```python
from build123d import *

# Parameters (mm, degrees)
SKETCH1_W           = 129.9464
SKETCH1_H           = 120.8024
BOSS_EXTRUDE1_DEPTH = 5.7912
SKETCH3_W           = 43.315466666
SKETCH3_H           = 5.7912
CUT_EXTRUDE2_DEPTH  = 89.900841825
SKETCH6_W           = 5.7912
SKETCH6_H           = 40.267466666
CUT_EXTRUDE5_DEPTH  = 89.900841825
SKETCH7_W           = 13.7668
SKETCH7_H           = 2.6035
CUT_EXTRUDE6_DEPTH  = 89.900841825
SKETCH8_W           = 2.0828
SKETCH8_H           = 6.1722
CUT_EXTRUDE7_DEPTH  = 89.900841825
CAVITY1_START       = -64.9732
CAVITY1_OUTLINE_W   = 40.267466667
CAVITY1_OUTLINE_H   = 5.7912
CAVITY1_DEPTH       = 5.7912
CAVITY1_START_2     = 21.657733333
CAVITY1_2_OUTLINE_W = 5.7912
CAVITY1_2_OUTLINE_H = 5.7912
CAVITY1_2_DEPTH     = 43.315466667
CAVITY1_START_3     = -59.182
CAVITY1_3_OUTLINE_W = 5.7912
CAVITY1_3_OUTLINE_H = 5.7912
CAVITY1_3_DEPTH     = 37.524266667


# Read off the part's stored shape, not the designer's step: Cavity1
with BuildPart() as part:
    # Sketch1 → Boss-Extrude1 (new body)
    with BuildSketch(Plane.XY):
        Rectangle(SKETCH1_W, SKETCH1_H)
    extrude(amount=BOSS_EXTRUDE1_DEPTH)

    # Sketch3 → Cut-Extrude2 (cut, through all)
    with BuildSketch(Plane(origin=(0, 0, 0), x_dir=(-1, 0, 0), z_dir=(0, 0, -1))):
        with Locations((0, -57.5056)):
            Rectangle(SKETCH3_W, SKETCH3_H)
    extrude(amount=-CUT_EXTRUDE2_DEPTH, mode=Mode.SUBTRACT)

    # Sketch6 → Cut-Extrude5 (cut, through all)
    with BuildSketch(Plane(origin=(0, 0, 0), x_dir=(-1, 0, 0), z_dir=(0, 0, -1))):
        with Locations((-62.0776, 0)):
            Rectangle(SKETCH6_W, SKETCH6_H)
    extrude(amount=-CUT_EXTRUDE5_DEPTH, mode=Mode.SUBTRACT)

    # Sketch7 → Cut-Extrude6 (cut, through all)
    with BuildSketch(Plane(origin=(0, 0, 0), x_dir=(-1, 0, 0), z_dir=(0, 0, -1))):
        with Locations((-52.2986, 0)):
            Rectangle(SKETCH7_W, SKETCH7_H)
    extrude(amount=-CUT_EXTRUDE6_DEPTH, mode=Mode.SUBTRACT)

    # Sketch8 → Cut-Extrude7 (cut, through all)
    with BuildSketch(Plane(origin=(0, 0, 0), x_dir=(-1, 0, 0), z_dir=(0, 0, -1))):
        with Locations((-52.2986, 0)):
            Rectangle(SKETCH8_W, SKETCH8_H)
    extrude(amount=-CUT_EXTRUDE7_DEPTH, mode=Mode.SUBTRACT)

    # Cavity1 outline → Cavity1 (cut)
    with BuildSketch(Plane.YZ.offset(CAVITY1_START)):
        with Locations((40.267466666, 2.8956)):
            Rectangle(CAVITY1_OUTLINE_W, CAVITY1_OUTLINE_H)
        with Locations((-40.267466666, 2.8956)):
            Rectangle(CAVITY1_OUTLINE_W, CAVITY1_OUTLINE_H)
    extrude(amount=CAVITY1_DEPTH, mode=Mode.SUBTRACT)

    # Cavity1 2 outline → Cavity1 2 (cut)
    with BuildSketch(Plane.YZ.offset(CAVITY1_START_2)):
        with Locations((57.5056, 2.8956)):
            Rectangle(CAVITY1_2_OUTLINE_W, CAVITY1_2_OUTLINE_H)
    extrude(amount=CAVITY1_2_DEPTH, mode=Mode.SUBTRACT)

    # Cavity1 3 outline → Cavity1 3 (cut)
    with BuildSketch(Plane.YZ.offset(CAVITY1_START_3)):
        with Locations((57.5056, 2.8956)):
            Rectangle(CAVITY1_3_OUTLINE_W, CAVITY1_3_OUTLINE_H)
    extrude(amount=CAVITY1_3_DEPTH, mode=Mode.SUBTRACT)


solid = part.part
```
Could you check a few things on this model? Use its own coordinates, in mm. A direction names the side the tool comes from. Round coordinates to 2 decimals unless told otherwise and drop trailing zeros. Loops run counter-clockwise (first coordinate to the right, second up) from the corner with the lowest first, then second, coordinate; pieces in that order, holes last. Notation, with made-up numbers: (24, 78) -> (36, 78) arc R20 cw to (36, 111) -> close; hole circle Ø4 at (-12.5, 38). An arc over 180 degrees is marked (long way). One line per question, with ' | ' between items.
(1) If I drill on probe 1 along X at (y, z) = (49, 4.4); probe 2 along Y at (x, z) = (-51.5, 4.8); probe 3 along Y at (x, z) = (-18, 1.6), over which ranges is the centre line in solid material (lowest first)?
Model answer:
probe 1: x = -59.18 to 64.97 | probe 2: y = -60.4 to 54.61 | probe 3: y = -54.61 to 60.4
(2) For pin 1 Ø1.7 at (x, z) = (-46.5, 2) entering from +Y; pin 2 Ø1.7 at (x, z) = (-62.5, 1.5) entering from -Y; pin 3 Ø8 at (x, y) = (-47.5, 21) entering from -Z; pin 4 Ø3 at (y, z) = (37.5, 3.5) entering from -X, each with a flat end and sliding along its axis, tell me the tip position at first contact or that it passes through.
Model answer:
pin 1: stops at y = 54.61 | pin 2: stops at y = -20.13 | pin 3: stops at z = 0 | pin 4: stops at x = -59.18
(3) Thinking about a two-plate mould opening in X: for faces 4 (the face through (-64.973, 0, 3)), 5 (the face through (-1, 1, 5.791)), 6 (the face through (64.973, 37, 3)), 7 (the face through (21.658, -58, 3)), which applies, released by +X, released by -X, zero draft, split by the parting line, or undercut?
Model answer:
face 4: released by -X | face 5: zero draft | face 6: released by +X | face 7: undercut
(4) If we section it at B-B on x = 36: List the corners of the cut face in (y, z) for me.
Model answer:
outline: (-60.4, 0) -> (54.61, 0) -> (54.61, 5.79) -> (-60.4, 5.79) -> close
(5) For faces 1 (the face through (-41, 54.61, 3)), 2 (the face through (0, -54.61, 3)), 3 (the face through (62, 20.134, 3)), which set-ups out of +Z, -Z, +X, -X, +Y, -Y let a thin tool reach every point of the face, with its end or its side?
Model answer:
face 1: +Z, -Z, -X, +Y | face 2: +Z, -Z, -Y | face 3: +Z, -Z, +X
(6) If we section it at C-C on y = 48: List the corners of the cut face in (x, z) for me, and give its area (3 significant figures).
Model answer:
outline: (-59.18, 0) -> (64.97, 0) -> (64.97, 5.79) -> (-59.18, 5.79) -> close | area: 719 mm^2
